CAD build for the part. Positions are in the model's coordinates, mm. A direction names the side the tool comes from. Round coordinates to 2 decimals unless told otherwise and drop trailing zeros. Loops run counter-clockwise (first coordinate to the right, second up) from the corner with the lowest first, then second, coordinate; pieces in that order, holes last. Notation, with made-up numbers: M 23,61.5 L 42,61.5 A23 cw 42,99.5 Z; hole C 70.5,-8.75 d3. An arc over 180 degrees is marked long. One line per item, written item: value. Start each with the question number.
Autodesk Inventor part; units mm, degrees
ref_plane "YZ Plane" through (0, 0, 0) normal (1, 0, 0) x (0, 1, 0)
ref_plane "XZ Plane" through (0, 0, 0) normal (0, 1, 0) x (-1, 0, 0)
ref_plane "XY Plane" through (0, 0, 0) normal (0, 0, 1) x (1, 0, 0)
sketch "Sketch1" plane through (0, 0, 0) normal (0, 1, 0) x (-1, 0, 0)
  line L0 (6, 19) -> (6, -19)
  line L1 (6, -19) -> (-6, -19)
  line L2 (-6, -19) -> (-6, 19)
  line L3 (-6, 19) -> (6, 19)
  line L4 (6, 19) -> (-6, -19) construction
  line L5 (6, -19) -> (-6, 19) construction
  point P0 (0, 0)
  dimension "d0" = 38
  dimension "d1" = 12
extrude "Extrusion1" add sketch "Sketch1" along normal blind 1
sketch "Sketch2" plane through (0, 1, 0) normal (0, 1, 0) x (1, 0, 0)
  point P0 (0, 0)
sketch "Sketch3" plane through (0, 1, 0) normal (0, 1, 0) x (1, 0, 0)
  line L0 (-6, -14) -> (-6, 16)
  line L1 (-6, 16) -> (6, 16)
  line L2 (6, 16) -> (6, -14)
  line L3 (6, -14) -> (-6, -14)
  line L4 (-6, -14) -> (6, 16) construction
  line L5 (-6, 16) -> (6, -14) construction
  line L6 (-6, -19) -> (6, -19)
  line L7 (-6, 19) -> (-6, -19)
  line L8 (-6, 16) -> (-6, 19)
  dimension "d4" = 30
  dimension "d5" = 12
extrude "Extrusion2" add sketch "Sketch3" along normal blind 1
sketch "Sketch4" plane through (0, 2, 0) normal (0, 1, 0) x (1, 0, 0)
  point P0 (0, 0)
sketch "Sketch5" plane through (0, 2, 0) normal (0, 1, 0) x (1, 0, 0)
  point P0 (0, 0)
sketch "Sketch6" plane through (0, 0, 0) normal (0, -1, 0) x (1, 0, 0)
  line L0 (-6, 19) -> (6, 19)
  line L1 (0, 19) -> (5, 19)
  line L2 (-5, 17) -> (-5, 19)
  line L3 (-5, 19) -> (5, 19)
  line L4 (5, 19) -> (5, 17)
  line L5 (5, 17) -> (-5, 17)
  point P0 (0, 0)
  dimension "d11" = 5
  dimension "d12" = 2
  dimension "d13" = 5
extrude "Extrusion3" add sketch "Sketch6" along normal blind 2
sketch "Sketch7" plane through (0, -2, 0) normal (0, -1, 0) x (1, 0, 0)
  circle A0 centre (0, 18.0182) radius 0.5
  circle A1 centre (-3.7835, 18) radius 0.5
  circle A2 centre (2.8577, 18) radius 0.5
  point P0 (0, 0)
  dimension "d16" = 1
  dimension "d17" = 1
  dimension "d18" = 1
extrude "Extrusion4" add sketch "Sketch7" along normal blind 5
sketch "Sketch8" plane through (0, 2, 0) normal (0, 1, 0) x (1, 0, 0)
  line L0 (-6, -14) -> (6, -14)
  line L1 (-4, -12) -> (-4, 11)
  line L2 (-4, 11) -> (2, 11)
  line L3 (2, 11) -> (2, -12)
  line L4 (2, -12) -> (-4, -12)
  point P0 (0, 0)
  dimension "d31" = 23
  dimension "d32" = 6
extrude "Extrusion5" add sketch "Sketch8" along normal blind 0.5
properties part number "OLED_128x32"
(1) Flat gauge pins, fed straight in: P1, Ø0.6, axis at y = -1.5, z = 18.5, coming from the +X side; P2, Ø1, axis at x = -4, z = 9, coming from the -Y side; P3, Ø1.6, axis at y = -0.5, z = 18.5, coming from the -X side; P4, Ø0.9, axis at x = -2.5, z = -17, coming from the +Y side. Where does each tip first touch, or does it go through?
(2) Mould opens along X. For faces 5 (the flat face through (6, 1, 0)), 6 (the cylindrical face through (0.269, -4.465, 17.597)), 7 (the flat face through (0, -7, 18)) say: pulls with the +X half, pulls with the -X half, needs draft (parallel to the pull), parting line crosses it, or undercut.
(3) Slice it at B-B, the plane z = -10. List the corners of the cut face in (x, y), and give its area (3 significant figures).
(4) Slice it at C-C, the plane y = -2.5. List the corners of the cut face in (x, z), and give its area (3 significant figures).
(5) Which spindle directions (+Z, -Z, +X, -X, +Y, -Y) get a long thin tool onto all of the face, cutting with end or side? Do faces 1 (the flat face through (-0.1, 1.5, -16)), 2 (the flat face through (0, -1, 17)), 3 (the flat face through (-5, -1, 18)), 4 (the flat face through (5, -1, 18)). Say none if no direction does.
(6) Slice it at A-A, the plane x = 0. List the corners of the cut face in (y, z).
(7) Probe L1, parallel to Z at x = -4.75, y = -1; L2, parallel to Y at x = -0.75, z = -14; L3, parallel to Z at x = -4.5, y = 1.75. List the from-to ranges inside material, lowest first.
Check result:
1. P1: stops at x = 5
1. P2: stops at y = 0
1. P3: stops at x = -6
1. P4: stops at y = 1
2. face 5: pulls with the +X half
2. face 6: undercut
2. face 7: needs draft
3. outline: M -6,0 L 6,0 L 6,2 L 2,2 L 2,2.5 L -4,2.5 L -4,2 L -6,2 Z
3. area: 27.0 mm^2
4. outline: C -3.78,18 d1; C 0,18.02 d1; C 2.86,18 d1
4. area: 2.36 mm^2
5. face 1: -Z, +X, -X, +Y
5. face 2: -Z, +X, -X, -Y
5. face 3: +Z, -Z, -X, -Y
5. face 4: +Z, -Z, +X, -Y
6. outline: M -7,17.52 L -2,17.52 L -2,17 L 0,17 L 0,-19 L 1,-19 L 1,-16 L 2,-16 L 2,-11 L 2.5,-11 L 2.5,12 L 2,12 L 2,14 L 1,14 L 1,19 L -2,19 L -2,18.52 L -7,18.52 Z
7. L1: z = 17 to 19
7. L2: y = 0 to 2
7. L3: z = -16 to 14
